Check sheet for the modelled part. Datum: model origin and axes. Units: mm. A direction names the side the tool comes from. Give positions to 0.01 mm unless a question says otherwise; leave off trailing zeros. Loops run counter-clockwise (first coordinate to the right, second up) from the corner with the lowest first, then second, coordinate; pieces in that order, holes last. Notation, with made-up numbers: (67.25, 14) - (110.25, 14) arc R19 ccw to (110.25, 49) - close; hole circle Ø11 at (-34, -7.75). An arc over 180 degrees is marked (long way). Answer in a Markdown table with one row per item. Add a question column.
(1) Go/stop test with flat-tipped pins: P1, Ø4, axis at x = 1.5, z = 4.5, coming from the +Y side; P2, Ø3, axis at x = 0, y = 6.5, coming from the +Z side; P3, Ø2, axis at x = -0.5, z = 3.5, coming from the -Y side. Record where each tip stops, or that it passes through.
(2) Draft check along X on faces 3 (the face through (4.565, 3.642, 3.633)), 4 (the face through (-6.199, 14.006, 3.597)), 5 (the face through (5.645, 2.33, 3.764)). Enter one of: released by +X, released by -X, zero draft, split by the parting line, or undercut.
(3) Thickness scan on L1, parallel to X at y = 10.5, z = 1; L2, parallel to X at y = 14.75, z = 6.5; L3, parallel to Y at x = 2, z = 3.75. Record the ranges inside material, lowest first.
(4) Sectioned sample at A-A on y = 11.5. Enter the section's corners in (x, z), then the cut area to 3 significant figures.
(5) Set-up check for faces 1 (the face through (1, 4, 7.236)), 2 (the face through (-5.096, 14.029, 3.567)): record each of +Z, -Z, +X, -X, +Y, -Y from which the full face is reachable in a straight line by a thin tool's end or side.
(6) Sectioned sample at B-B on x = 3. Enter the section's corners in (y, z), then the cut area to 3 significant figures.
from build123d import *

# Parameters (mm, degrees)
F1_DEPTH = 6.5
F2_DEPTH = 4.85
F3_R     = 1
F4_SIZE  = 0.5
F5_R     = 3


with BuildPart() as f1:
    # F0 (on Right) → F1 (new body, symmetric)
    with BuildSketch(Plane.YZ):
        Polygon((4.633555, 7.235633), (2, 0), (13, 0), (15.633555, 7.235633), align=None)
        Polygon((2.633555, 7.235633), (0, 0), (2, 0), (4.633555, 7.235633), align=None)
    extrude(amount=F1_DEPTH, both=True)

    # F0 (on Right) → F2 (cut, symmetric)
    with BuildSketch(Plane.YZ):
        Polygon((4.633555, 7.235633), (2, 0), (13, 0), (15.633555, 7.235633), align=None)
    extrude(amount=F2_DEPTH, both=True, mode=Mode.SUBTRACT)

    # F3
    f3_edges = [f1.edges().sort_by_distance(p)[0] for p in [
        (4.85, 3.316778, 3.617817),
        (-4.85, 3.316778, 3.617817),
        (-6.5, 14.316778, 3.617817),
        (6.5, 14.316778, 3.617817),
    ]]
    fillet(f3_edges, radius=F3_R)

    # F4
    f4_edges = [f1.edges().sort_by_distance(p)[0] for p in [
        (4.85, 14.316778, 3.617817),
        (-4.85, 14.316778, 3.617817),
    ]]
    chamfer(f4_edges, length=F4_SIZE)

    # F5
    f5_edges = [f1.edges().sort_by_distance(p)[0] for p in [
        (6.5, 1.316778, 3.617817),
        (-6.5, 1.316778, 3.617817),
    ]]
    fillet(f5_edges, radius=F5_R)


solid = f1.part
Reply:
| question | item | result |
|---|---|---|
| 1 | P1 | y = 4.37 |
| 1 | P2 | through |
| 1 | P3 | y = 0.91 |
| 2 | face 3 | undercut |
| 2 | face 4 | released by -X |
| 2 | face 5 | released by +X |
| 3 | L1 | -6.5 to -4.85, 4.85 to 6.5 |
| 3 | L2 | -6.41 to -4.85, 4.85 to 6.41 |
| 3 | L3 | 1.36 to 3.36 |
| 4 | outline | (-6.5, 0) - (-4.85, 0) - (-4.85, 7.24) - (-6.5, 7.24) - close; (4.85, 0) - (6.5, 0) - (6.5, 7.24) - (4.85, 7.24) - close |
| 4 | area | 23.9 mm^2 |
| 5 | face 1 | +Z, +X, -X, +Y, -Y |
| 5 | face 2 | -Z, +Y |
| 6 | outline | (0, 0) - (2, 0) - (4.63, 7.24) - (2.63, 7.24) - close |
| 6 | area | 14.5 mm^2 |
